Autodesk Inventor part; units mm, degrees
ref_plane "YZ Plane" through (0, 0, 0) normal (1, 0, 0) x (0, 1, 0)
ref_plane "XZ Plane" through (0, 0, 0) normal (0, 1, 0) x (-1, 0, 0)
ref_plane "XY Plane" through (0, 0, 0) normal (0, 0, 1) x (1, 0, 0)
sketch "Sketch1" plane through (0, 0, 0) normal (0, 0, 1) x (1, 0, 0)
  line L0 (0, 0) -> (10, 0)
  line L1 (0, 0) -> (0, 6.945) construction
  line L2 (0, 6.945) -> (0.5, 6.945)
  line L3 (0.5, 6.945) -> (0.5, 7.987)
  line L4 (0.5, 7.987) -> (4.82, 7.987)
  line L5 (5.12, 8.287) -> (5.12, 9.77)
  line L6 (5.12, 9.77) -> (2.695, 12.195)
  line L7 (2.695, 12.195) -> (0.275, 9.775)
  line L8 (0.275, 9.775) -> (0.275, 9.375)
  line L9 (0.275, 9.375) -> (0, 9.375)
  line L10 (4.82, 7.987) -> (5.12, 8.287)
  line L11 (0, 6.945) -> (0, 11.2763) construction
  line L12 (0, 6.945) -> (-0.5, 6.945)
  line L13 (-0.5, 6.945) -> (-0.5, 7.987)
  line L14 (-0.5, 7.987) -> (-4.82, 7.987)
  line L15 (-5.12, 8.287) -> (-5.12, 9.77)
  line L16 (-5.12, 9.77) -> (-2.695, 12.195)
  line L17 (-2.695, 12.195) -> (-0.275, 9.775)
  line L18 (-0.275, 9.775) -> (-0.275, 9.375)
  line L19 (-0.275, 9.375) -> (0, 9.375)
  line L20 (-4.82, 7.987) -> (-5.12, 8.287)
  point P0 (5.12, 7.987)
  point P1 (-5.12, 7.987)
  dimension "d0" = 10
  dimension "d2" = 0.5
  dimension "d3" = 15.974
  dimension "d4" = 13.89
  dimension "d5" = 0.3
  dimension "d6" = 0.3
  dimension "d7" = 19.54
  dimension "d8" = 5.12
  dimension "d12" = 24.39
  dimension "d14" = 18.75
  dimension "d16" = 0.275
  dimension "d17" = 135
  dimension "d18" = 135
  dimension "d19" = 2.695
revolve "Revolution1" add sketch "Sketch1" angle 360 about axis through (0, 0, 0) along (1, 0, 0)
properties part number "Dual V Wheel" material "Acetal Resin, Black"
Verification items for the finished model (mm, model axes). A direction names the side the tool comes from. Coordinates: 2 decimals unless noted, no trailing zeros. Loops run counter-clockwise (first coordinate to the right, second up) from the corner with the lowest first, then second, coordinate; pieces in that order, holes last. Notation, with made-up numbers: (16, -0.75) -> (75, -0.75) arc R25 cw to (75, 30.25) -> close; hole circle Ø7 at (43, 76). An arc over 180 degrees is marked (long way). Answer in a Markdown table with one row per item. Add a question column.
1. Depth check by flat-ended pin: P1, Ø6, axis at y = -0.5, z = 4, coming from the -X side; P2, Ø2, axis at x = 0, y = -5, coming from the +Z side; P3, Ø3, axis at y = -7, z = 9, coming from the -X side. Enter the tip coordinate at first touch or a pass-through.
2. Section check D-D, the plane x = -1.75. Enter the section's corners in (y, z), then the cut area to 3 significant figures.
3. Access from +Z, -Z, +X, -X, +Y, -Y to the whole of each face (thin tool, end or side, straight path). Record for faces 4 (the face through (0.5, -2, 7)), 5 (the face through (-2.69, -5.887, -5.398)), 6 (the face through (-0.426, -2.152, 9.69)), 7 (the face through (5.12, -4.4, -7.2)).
4. Material ranges on probe 1 along Z at (x, y) = (0, 0) (3 decimals); probe 2 along X at (y, z) = (-4.5, 5.75); probe 3 along Z at (x, y) = (-2.6, 0), recorded low to high. Write a range as [from, to].
5. Section check C-C, the plane x = -3.75. Enter the section's corners in (y, z).
6. Draft check along Z on faces 1 (the face through (0.01, -1.51, -6.78)), 2 (the face through (0.004, -1.22, 9.295)), 3 (the face through (-5.12, -4.4, -7.2)). Enter one of: +Z half, -Z half, draft (parallel to the pull), parting line (faces both ways), or undercut.
Derived:
| question | item | result |
|---|---|---|
| 1 | P1 | stops at x = -0.5 |
| 1 | P2 | stops at z = 9.35 |
| 1 | P3 | stops at x = -4.99 |
| 2 | outline | circle Ø22.5 at (0, 0); hole circle Ø15.97 at (0, 0) |
| 2 | area | 197 mm² |
| 3 | face 4 | +X |
| 3 | face 5 | -X |
| 3 | face 6 | none |
| 3 | face 7 | +Z, -Z, +X, +Y, -Y |
| 4 | probe 1 | z = [-9.375, -6.945], [6.945, 9.375] |
| 4 | probe 2 | x = [-0.5, 0.5] |
| 4 | probe 3 | z = [-12.1, -7.99], [7.99, 12.1] |
| 5 | outline | circle Ø22.28 at (0, 0); hole circle Ø15.97 at (0, 0) |
| 6 | face 1 | undercut |
| 6 | face 2 | parting line |
| 6 | face 3 | draft |
